```python
from build123d import *

# Parameters (mm, degrees)
F0_W      = 180
F0_H      = 30
F0_R      = 1
F0_W_2    = 100
F0_H_2    = 16
F1_DEPTH  = 5
F2_R      = 12.5
F2_R_2    = 0.5
F2_R_3    = 2.75
F3_DEPTH  = 3
F4_DEPTH  = 25
F5_R      = 14.99999
F2_R_4    = 5
F6_DEPTH  = 25
F7_R      = 5
F2_W      = 14
F2_H      = 18
F8_DEPTH  = 20
F9_R      = 6
F2_R_5    = 1
F10_DEPTH = 2
F11_W     = 6
F11_H     = 14
F12_DEPTH = 25
F13_R     = 2
F15_DEPTH = 25


# Not quite as in the source:
# - a fillet or chamfer is up to 0.001 mm smaller than in the source, because OpenCascade refuses the exact size


with BuildPart() as f1:
    # F0 (on Top) → F1 (new body)
    with BuildSketch(Plane.XY):
        with Locations((10, -11.8972941886)):
            Rectangle(F0_W, F0_H)
        with Locations((-76, -22.8972941886)):
            Circle(F0_R, mode=Mode.SUBTRACT)
        with Locations((14.5, -23.3972941886)):
            Circle(F0_R, mode=Mode.SUBTRACT)
        with Locations((10, -11.8972941886)):
            Rectangle(F0_W_2, F0_H_2, mode=Mode.SUBTRACT)
        with Locations((65, -18.6472941886)):
            Circle(F0_R, mode=Mode.SUBTRACT)
        with Locations((-76, -0.8972941886)):
            Circle(F0_R, mode=Mode.SUBTRACT)
        with Locations((65, -5.1472941886)):
            Circle(F0_R, mode=Mode.SUBTRACT)
        with Locations((14.5, -0.3972941886)):
            Circle(F0_R, mode=Mode.SUBTRACT)
    extrude(amount=F1_DEPTH)

    # F2 (on face) → F3 (cut)
    with BuildSketch(Plane.XY.offset(5)):
        with Locations((85, -11.8972941886)):
            Circle(F2_R)
        with Locations((85, -20.8972941886)):
            Circle(F2_R_2, mode=Mode.SUBTRACT)
        with Locations((85, -11.8972941886)):
            Circle(F2_R_3, mode=Mode.SUBTRACT)
        with Locations((77, -11.8972941886)):
            Circle(F2_R_2, mode=Mode.SUBTRACT)
        with Locations((93, -11.8972941886)):
            Circle(F2_R_2, mode=Mode.SUBTRACT)
        with Locations((85, -2.8972941886)):
            Circle(F2_R_2, mode=Mode.SUBTRACT)
    extrude(amount=-F3_DEPTH, mode=Mode.SUBTRACT)

    # F2 (on face) → F4 (cut)
    with BuildSketch(Plane.XY.offset(5)):
        with Locations((85, -11.8972941886)):
            Circle(F2_R_3)
        with Locations((85, -2.8972941886)):
            Circle(F2_R_2)
        with Locations((77, -11.8972941886)):
            Circle(F2_R_2)
        with Locations((85, -20.8972941886)):
            Circle(F2_R_2)
        with Locations((93, -11.8972941886)):
            Circle(F2_R_2)
    extrude(amount=-F4_DEPTH, mode=Mode.SUBTRACT)

    # F5 (radius 15 in the source; OpenCascade refuses exactly that, so slightly less here)
    f5_edges = [f1.edges().sort_by_distance(p)[0] for p in [
        (100, 3.102706, 2.5),
        (100, -26.897294, 2.5),
    ]]
    fillet(f5_edges, radius=F5_R)

    # F2 (on face) → F6 (cut)
    with BuildSketch(Plane.XY.offset(5)):
        with Locations((-65, -11.8972941886)):
            Circle(F2_R_4)
    extrude(amount=-F6_DEPTH, mode=Mode.SUBTRACT)

    # F7
    f7_edges = [f1.edges().sort_by_distance(p)[0] for p in [
        (-40, -3.897294, 2.5),
        (-40, -19.897294, 2.5),
        (60, -3.897294, 2.5),
        (60, -19.897294, 2.5),
    ]]
    fillet(f7_edges, radius=F7_R)

    # F2 (on face) → F8 (join)
    with BuildSketch(Plane.XY.offset(5)):
        with Locations((-65, -10.8972941886)):
            Rectangle(F2_W, F2_H)
        with Locations((-65, -11.8972941886)):
            Circle(F2_R_4, mode=Mode.SUBTRACT)
    extrude(amount=F8_DEPTH)

    # F9
    f9_edges = [f1.edges().sort_by_distance(p)[0] for p in [
        (-72, -19.897294, 15),
        (-58, -19.897294, 15),
        (-72, -1.897294, 15),
        (-58, -1.897294, 15),
    ]]
    fillet(f9_edges, radius=F9_R)

    # F2 (on face) → F10 (cut)
    with BuildSketch(Plane.XY.offset(5)):
        Polygon((-72, -19.8972941886), (-72, -1.8972941886), (-72, 3.1027058114), (-80, 3.1027058114), (-80, -26.8972941886), (-72, -26.8972941886), align=None)
        with Locations((-76, -22.8972941886)):
            Circle(F2_R_5, mode=Mode.SUBTRACT)
        with Locations((-76, -0.8972941886)):
            Circle(F2_R_5, mode=Mode.SUBTRACT)
    extrude(amount=-F10_DEPTH, mode=Mode.SUBTRACT)

    # F11 (on face) → F12 (cut)
    with BuildSketch(Plane.YZ.offset(-58)):
        with Locations((-10.8972941886, 15)):
            Rectangle(F11_W, F11_H)
    extrude(amount=-F12_DEPTH, mode=Mode.SUBTRACT)

    # F13
    f13_edges = [f1.edges().sort_by_distance(p)[0] for p in [
        (-59.208712, -13.897294, 8),
        (-60, -7.897294, 8),
        (-60, -7.897294, 22),
        (-59.208712, -13.897294, 22),
        (-70.791288, -13.897294, 8),
        (-70, -7.897294, 8),
        (-70, -7.897294, 22),
        (-70.791288, -13.897294, 22),
    ]]
    fillet(f13_edges, radius=F13_R)

    # F14 (on face) → F15 (cut)
    with BuildSketch(Plane(origin=(0, -1.8972941886, 0), x_dir=(-1, 0, 0), z_dir=(0, 1, 0))):
        with BuildLine():
            ThreePointArc((64, 20), (65, 19), (66, 20))
            ThreePointArc((66, 20), (65, 21), (64, 20))
        make_face()
        with BuildLine():
            ThreePointArc((64, 14), (65, 13), (66, 14))
            ThreePointArc((66, 14), (65, 15), (64, 14))
        make_face()
    extrude(amount=-F15_DEPTH, mode=Mode.SUBTRACT)


solid = f1.part
```
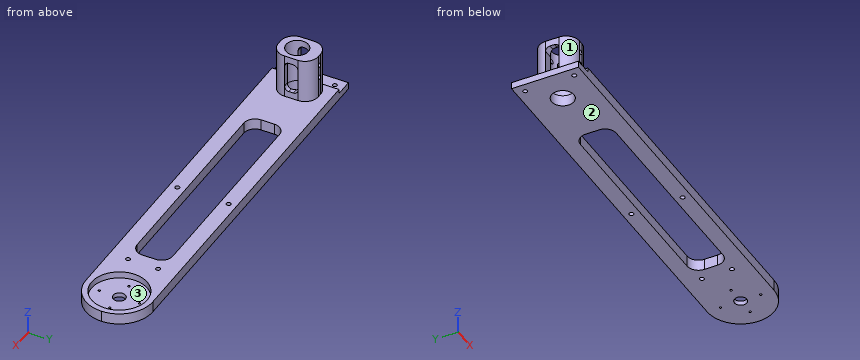
Here's how the part is built. I have some questions about the finished solid (model axes, mm). Face numbers are marked on the shaded views. Coordinates: 2 decimals unless noted, no trailing zeros. Order: outer loops, then holes, each group sorted by start corner. A loop starts at its lowest first (then second) coordinate and runs counter-clockwise, first axis right, second up. Notation, with made-up numbers: (-17, -4) - (8, -4) arc R30 cw to (8, 35) - close; hole circle Ø10 at (34, -5.75). An arc over 180 degrees is marked (long way). One line per question, with ' | ' between items. Start each with the question number.
1. If we section it at B-B (x = -17): Write out the boundary of the cut face in (y, z).
2. Please list where these lines run through material, in increasing order: line 1 along Z through (x, y) = (-65, -17); line 2 along Y through (x, z) = (14.5, 3.45); line 3 along X through (y, z) = (-6, 3.75) (3 decimals). Write a range as [from, to].
3. If we mould it in two halves opening along Y, with no side actions, what happens to the marked faces 1, 2 and 3? For each: released by +Y, released by -Y, zero draft, split by the parting line, or undercut.
4. If we section it at C-C (x = -38.5): Write out the boundary of the cut face in (y, z).
5. I'm going to push flat-ended pins straight in: pin 1 Ø1 at (x, z) = (-3, 6.5) entering from -Y; pin 2 Ø3 at (y, z) = (-7.5, 10.5) entering from +X; pin 3 Ø2.5 at (x, z) = (-65, 20) entering from -Y; pin 4 Ø0.6 at (x, z) = (-65, 11.5) entering from +Y. Where does each tip first touch, or does it pass through?
6. If we section it at A-A (z = 17.5): Write out the boundary of the cut face in (x, y), and give its area (3 significant figures).
Model answer:
1) outline: (-26.9, 0) - (-19.9, 0) - (-19.9, 5) - (-26.9, 5) - close; (-3.9, 0) - (3.1, 0) - (3.1, 5) - (-3.9, 5) - close
2) line 1: z = [0, 13], [15, 19], [21, 25] | line 2: y = [-26.9, -24.4], [-22.4, -19.9], [-3.9, -1.4], [0.6, 3.1] | line 3: x = [-72, -39.075], [59.075, 64.478], [65.522, 73.979], [96.021, 98.792]
3) face 1: released by -Y | face 2: zero draft | face 3: undercut
4) outline: (-26.9, 0) - (-18.47, 0) - (-18.47, 5) - (-26.9, 5) - close; (-5.33, 0) - (3.1, 0) - (3.1, 5) - (-5.33, 5) - close
5) pin 1: passes through | pin 2: stops at x = -58 | pin 3: stops at y = -19.9 | pin 4: stops at y = -1.9
6) outline: (-72, -13.9) arc R6 ccw to (-66, -19.9) - (-64, -19.9) arc R6 ccw to (-58, -13.9) - (-60.42, -13.9) arc R5 cw to (-69.58, -13.9) - close; (-72, -7.9) - (-68, -7.9) arc R5 cw to (-62, -7.9) - (-58, -7.9) arc R6 ccw to (-64, -1.9) - (-66, -1.9) arc R6 ccw to start | area: 113 mm²
